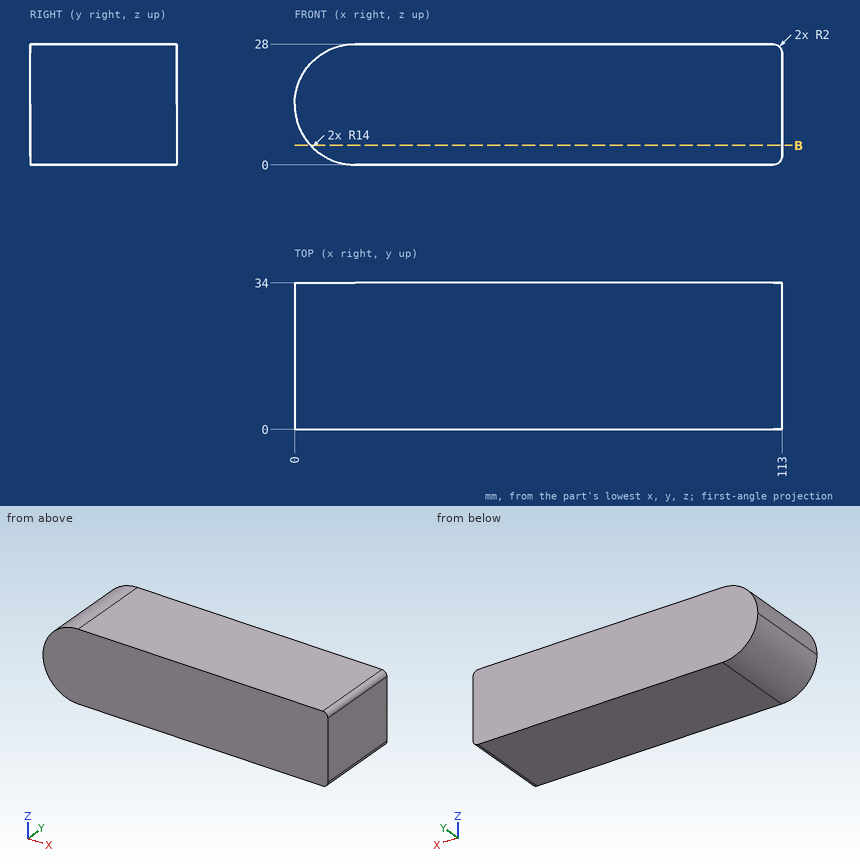
Input: dimensioned drawing with shaded views. Units: mm. Origin: part minimum x, y, z. Give positions to 0.01 mm unless a question says otherwise; leave off trailing zeros. Order: outer loops, then holes, each group sorted by start corner. A loop starts at its lowest first (then second) coordinate and runs counter-clockwise, first axis right, second up. Notation, with made-up numbers: (42.5, 29) -> (87.5, 29) arc R10 cw to (87.5, 39) -> close; hole circle Ø3 at (5.25, 2.25). An arc over 180 degrees is marked (long way). Answer as a JSON object with one key per item and string values.
Q1. Material intervals for probe 1 along X at (y, z) = (21, 14.5); probe 2 along X at (y, z) = (18.5, 10.25); probe 3 along Z at (x, y) = (10.5, 2), sorted ascending.
Entries:
{"probe 1": "x = 0.01 to 113", "probe 2": "x = 0.51 to 113", "probe 3": "z = 0.44 to 27.56"}
Q2. First-contact query: pin 1 (5 mm diameter, centred on y = 24, z = 21.5, fed in from -X); pin 2 (5 mm diameter, centred on y = 9.5, z = 20.5, fed in from -X). Flat tips, straight axial feed; report the tip coordinate or a pass-through.
Entries:
{"pin 1": "stops at x = 0.92", "pin 2": "stops at x = 0.58"}
Q3. Section B-B (z = 4.5). Output: boundary loops of the cut face in (x, y).
Entries:
{"outline": "(3.72, 0) -> (113, 0) -> (113, 34) -> (3.72, 34) -> close"}
